from build123d import *

# Parameters (mm, degrees)
SKETCH_1_R          = 4.15
EXTRUDE_1_DEPTH     = 20
SKETCH_2_R          = 4.923200542
EXTRUDE_2_DEPTH     = 3
SKETCH_3_R          = 1.25
CUT_EXTRUDE_1_DEPTH = 13


with BuildPart() as part:
    # Эскиз1 → Бобышка-Вытянуть1 (new body)
    with BuildSketch(Plane.XY):
        with BuildLine():
            Line((5.123475383, -4), (32.5, -4))
            Line((32.5, -4), (32.5, 0))
            Line((32.5, 0), (6.5, 0))
            ThreePointArc((6.5, 0), (-6.146242348, 2.115113473), (5.123475383, -4))
        make_face()
        Circle(SKETCH_1_R, mode=Mode.SUBTRACT)
    extrude(amount=EXTRUDE_1_DEPTH)

    # Эскиз2 → Бобышка-Вытянуть2 (add)
    with BuildSketch(Plane.XY.offset(20)):
        Circle(SKETCH_2_R)
    extrude(amount=-EXTRUDE_2_DEPTH)

    # Эскиз3 → Вырез-Вытянуть1 (cut)
    with BuildSketch(Plane(origin=(0, 0, 0), x_dir=(1, 0, 0), z_dir=(0, 1, 0))):
        with Locations((12.5, -5)):
            Circle(SKETCH_3_R)
        with Locations((28.5, -5)):
            Circle(SKETCH_3_R)
    extrude(amount=-CUT_EXTRUDE_1_DEPTH, mode=Mode.SUBTRACT)


solid = part.part
CAD build for the part. Positions are in the model's coordinates, mm. A direction names the side the tool comes from. Coordinates: 2 decimals unless noted, no trailing zeros. Loops run counter-clockwise (first coordinate to the right, second up) from the corner with the lowest first, then second, coordinate; pieces in that order, holes last. Notation, with made-up numbers: (29, 82) -> (67, 82) arc R15 cw to (67, 101) -> close; hole circle Ø3 at (74, 80). An arc over 180 degrees is marked (long way). One line per item, written item: value.
1. Which spindle directions (+Z, -Z, +X, -X, +Y, -Y) get a long thin tool onto all of the face, cutting with end or side? Do faces 1 (the face through (0, 0, 17)), 2 (the face through (32.5, -2, 10)), 3 (the face through (20, 0, 10)). Say none if no direction does.
Answers:
face 1: -Z
face 2: +Z, -Z, +X, +Y, -Y
face 3: +Z, -Z, +X, +Y
2. Flat gauge pins, fed straight in: P1, Ø5, axis at y = 4, z = 11.5, coming from the -X side; P2, Ø1.5, axis at y = -3.5, z = 8.5, coming from the -X side; P3, Ø4, axis at y = -2.5, z = 13, coming from the -X side. Where does each tip first touch, or does it go through?
Answers:
P1: stops at x = -6.32
P2: stops at x = -5.89
P3: stops at x = -6.48
3. Pull direction X, two halves, no side cores. Call faces 4 (the face through (19, -4, 10)), 5 (the face through (-0.9, -4.05, 8.38)), 6 (the face through (12.23, -1.97, 6.22)), 7 (the face through (-6.058, 2.355, 9.86)): pulls with the +X half, pulls with the -X half, needs draft (parallel to the pull), parting line crosses it, or undercut.
Answers:
face 4: needs draft
face 5: undercut
face 6: undercut
face 7: parting line crosses it
4. Slice it at B-B on z = 5. Write the cut outline in (x, y), and give its area (3 significant figures).
Answers:
outline: (5.12, -4) -> (11.25, -4) -> (11.25, 0) -> (6.5, 0) arc R6.5 ccw (long way) to start; (13.75, -4) -> (27.25, -4) -> (27.25, 0) -> (13.75, 0) -> close; (29.75, -4) -> (32.5, -4) -> (32.5, 0) -> (29.75, 0) -> close; hole circle Ø8.3 at (0, 0)
area: 164 mm^2
5. Drill centre lines: line 1 (Y direction, x = 0, z = 10.5); line 2 (X direction, y = -2.85, z = 5); line 3 (Z direction, x = 12.5, y = -1.35). Where is each one in solid material? Low to high. Write a range as [from, to].
Answers:
line 1: y = [-6.5, -4.15], [4.15, 6.5]
line 2: x = [-5.84, -3.02], [3.02, 11.25], [13.75, 27.25], [29.75, 32.5]
line 3: z = [0, 3.75], [6.25, 20]
6. Slice it at D-D on z = 3. Write the cut outline in (x, y), and give its area (3 significant figures).
Answers:
outline: (5.12, -4) -> (32.5, -4) -> (32.5, 0) -> (6.5, 0) arc R6.5 ccw (long way) to start; hole circle Ø8.3 at (0, 0)
area: 184 mm^2
7. Slice it at C-C on y = 2.75. Write the cut outline in (x, z), and give its area (3 significant figures).
Answers:
outline: (-5.89, 0) -> (-3.11, 0) -> (-3.11, 17) -> (3.11, 17) -> (3.11, 0) -> (5.89, 0) -> (5.89, 20) -> (-5.89, 20) -> close
area: 130 mm^2
8. Slice it at A-A on x = 28.5. Write the cut outline in (y, z), and give its area (3 significant figures).
Answers:
outline: (-4, 0) -> (0, 0) -> (0, 3.75) -> (-4, 3.75) -> close; (-4, 6.25) -> (0, 6.25) -> (0, 20) -> (-4, 20) -> close
area: 70.0 mm^2
